Build history of the part. All positions in model axes, mm. Face numbers are marked on the shaded views. A direction names the side the tool comes from. Round coordinates to 2 decimals unless told otherwise and drop trailing zeros. Loops run counter-clockwise (first coordinate to the right, second up) from the corner with the lowest first, then second, coordinate; pieces in that order, holes last.
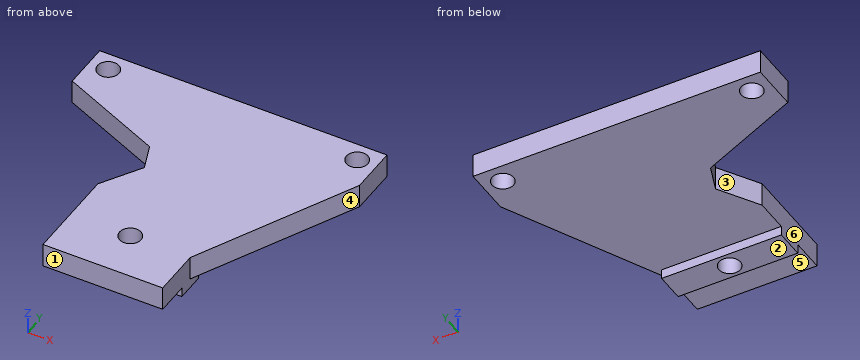
from build123d import *

# Parameters (mm, degrees)
BOSS_EXTRU_1_DEPTH      = 5
ESQUISSE2_W             = 25
ESQUISSE2_H             = 6
BOSS_EXTRU_2_DEPTH      = 2
ESQUISSE3_R             = 2.25
ENL_V_MAT_EXTRU_3_DEPTH = 8.1


with BuildPart() as part:
    # Esquisse1 → Boss.-Extru.1 (new body)
    with BuildSketch(Plane.XY):
        Polygon((0, 0), (60, 0), (60, -10), (38.522739923, -19.314739888), (36.355716988, -24.967843196), (41.356924968, -33.188115427), (41.356924968, -53.188115427), (16.356924968, -53.188115427), (16.356924968, -43.188115427), (0, -10), align=None)
    extrude(amount=BOSS_EXTRU_1_DEPTH)

    # Esquisse2 → Boss.-Extru.2 (add)
    with BuildSketch(Plane(origin=(0, 0, 0), x_dir=(-1, 0, 0), z_dir=(0, 0, -1))):
        with Locations((-28.856924968, -43.188115427)):
            Rectangle(ESQUISSE2_W, ESQUISSE2_H)
    extrude(amount=BOSS_EXTRU_2_DEPTH)

    # Esquisse3 → Enlèv. mat.-Extru.3 (cut)
    with BuildSketch(Plane(origin=(0, 0, -2), x_dir=(-1, 0, 0), z_dir=(0, 0, -1))):
        with Locations((-28.856924968, -43.188115427)):
            Circle(ESQUISSE3_R)
        with Locations(Location((-56, -3.88, 0), (0, 0, 180))):
            Circle(ESQUISSE3_R)
        with Locations(Location((-4, -3.88, 0), (0, 0, 180))):
            Circle(ESQUISSE3_R)
    extrude(amount=-ENL_V_MAT_EXTRU_3_DEPTH, mode=Mode.SUBTRACT)

    # Symétrie1: part across plane


with BuildPart() as part_1:
    add(part.part)
    add(part.part.mirror(Plane(origin=(0, 0, 5), x_dir=(0, 0, 1), z_dir=(1, 0, 0))))

    # Fractionner1
    split(bisect_by=Plane(origin=(0, 0, 0), x_dir=(0, 0, -1), z_dir=(-1, 0, 0)), keep=Keep.TOP)


solid = part_1.part
(1) Slice it at B-B on z = 3. List the corners of the cut face in (x, y).
Responses:
outline: (-60, -10) - (-38.52, -19.31) - (-36.36, -24.97) - (-41.36, -33.19) - (-41.36, -53.19) - (-16.36, -53.19) - (-16.36, -43.19) - (0, -10) - (0, 0) - (-60, 0) - close; hole circle Ø4.5 at (-56, -3.88); hole circle Ø4.5 at (-28.86, -43.19); hole circle Ø4.5 at (-4, -3.88)
(2) Pull direction Y, two halves, no side cores. Call the marked faces 1, 2 and 3: +Y half, -Y half, draft (parallel to the pull), parting line (faces both ways), or undercut.
Responses:
face 1: -Y half
face 2: draft
face 3: undercut
(3) Which spindle directions (+Z, -Z, +X, -X, +Y, -Y) get a long thin tool onto all of the face, cutting with end or side? Do the marked faces 4, 5 and 6. Say none if no direction does.
Responses:
face 4: +Z, -Z, +X, -Y
face 5: -Z, +X, -X, -Y
face 6: +Z, -Z, -X, -Y
(4) Slice it at A-A on y = -3.88. List the corners of the cut face in (x, z).
Responses:
outline: (-60, 0) - (-58.25, 0) - (-58.25, 5) - (-60, 5) - close; (-53.75, 0) - (-6.25, 0) - (-6.25, 5) - (-53.75, 5) - close; (-1.75, 0) - (0, 0) - (0, 5) - (-1.75, 5) - close
(5) Slice it at C-C on x = -4. List the corners of the cut face in (y, z), plus the area to 3 significant figures.
Responses:
outline: (-18.12, 0) - (-6.13, 0) - (-6.13, 5) - (-18.12, 5) - close; (-1.63, 0) - (0, 0) - (0, 5) - (-1.63, 5) - close
area: 68.1 mm2
(6) Slice it at D-D on x = -21.5. List the corners of the cut face in (y, z).
Responses:
outline: (-53.19, 0) - (-46.19, 0) - (-46.19, -2) - (-40.19, -2) - (-40.19, 0) - (0, 0) - (0, 5) - (-53.19, 5) - close
(7) Probe line 1 (X direction, y = -43, z = -1.25); line 2 (Z direction, x = -18.5, y = -22); line 3 (X direction, y = -44.5, z = 2.5). List the from-to ranges inside material, lowest first.
Responses:
line 1: x = -41.36 to -31.1, -26.61 to -16.36
line 2: z = 0 to 5
line 3: x = -41.36 to -30.68, -27.03 to -16.36
(8) Pin check, flat tips, straight feed: P1, Ø6, axis at x = -56, y = -3.88, coming from the -Z side; P2, Ø1, axis at x = -30.5, z = -1, coming from the +Y side; P3, Ø2, axis at y = -45.5, z = 3, coming from the +X side. Stop position of each tip, or through.
Responses:
P1: stops at z = 0
P2: stops at y = -40.19
P3: stops at x = -16.36
